from build123d import *

# Parameters (mm, degrees)
F0_W     = 127
F0_H     = 76.2
F1_DEPTH = 25.4
F2_W     = 123.0376
F2_H     = 72.2376
F3_DEPTH = 24.4094
F4_W     = 1.9812
F4_H     = 72.2376
F5_DEPTH = 24.4094
F6_W     = 21.4376
F6_H     = 72.2376
F7_DEPTH = 1.9812


with BuildPart() as f1:
    # F0 (on Front) → F1 (new body)
    with BuildSketch(Plane.XZ):
        Rectangle(F0_W, F0_H)
    extrude(amount=F1_DEPTH)

    # F2 (on Front) → F3 (cut)
    with BuildSketch(Plane.XZ):
        Rectangle(F2_W, F2_H)
    extrude(amount=F3_DEPTH, mode=Mode.SUBTRACT)

    # F4 (on face) → F5 (join)
    with BuildSketch(Plane(origin=(0, -24.4094, 0), x_dir=(-1, 0, 0), z_dir=(0, 1, 0))):
        with Locations((-43.5102, 0)):
            Rectangle(F4_W, F4_H)
    extrude(amount=F5_DEPTH)

    # F6 (on face) → F7 (cut)
    with BuildSketch(Plane(origin=(-63.5, 0, 0), x_dir=(0, -1, 0), z_dir=(-1, 0, 0))):
        with Locations((12.7, 0)):
            Rectangle(F6_W, F6_H)
    extrude(amount=-F7_DEPTH, mode=Mode.SUBTRACT)


solid = f1.part
Could you check a few things on this model? Use its own coordinates, in mm. A direction names the side the tool comes from. Give positions to 0.01 mm unless a question says otherwise; leave off trailing zeros. Order: outer loops, then holes, each group sorted by start corner. A loop starts at its lowest first (then second) coordinate and runs counter-clockwise, first axis right, second up. Notation, with made-up numbers: (79.25, 33) - (103.25, 33) arc R21 cw to (103.25, 60) - close; hole circle Ø1 at (81, 5.25). An arc over 180 degrees is marked (long way). One line per item, written item: value. Start each with the question number.
1. Thinking about a two-plate mould opening in Z: for faces 3 (the face through (-1, -13, -38.1)), 4 (the face through (53, -24.409, 1)), 5 (the face through (0, 0, 37)), 6 (the face through (-1, -13, 38.1)), which applies, +Z half, -Z half, draft (parallel to the pull), parting line (faces both ways), or undercut?
2. If I drill on probe 1 along Z at (x, y) = (-48.5, -19); probe 2 along X at (y, z) = (-11.75, 27); probe 3 along Y at (x, z) = (46.5, -6.5), over which ranges is the centre line in solid material (lowest first)?
3. Imagine slicing it at C-C on x = 36.5. List the corners of the cut face in (y, z) for me, plus the area to 3 significant figures.
4. Imagine slicing it at B-B on y = -20.25. List the corners of the cut face in (x, z) for me, plus the area to 3 significant figures.
5. For P1, Ø3, axis at y = -20.5, z = 15, coming from the -X side; P2, Ø13.5, axis at x = 53, z = -8.5, coming from the +Y side, each with a flat end and sliding along its axis, tell me the tip position at first contact or that it passes through.
6. Imagine slicing it at A-A on z = -27.5. List the corners of the cut face in (x, y) for me.
7. For faces 1 (the face through (-63.5, -24, -3)), 2 (the face through (61.519, -12, -1)), which set-ups out of +Z, -Z, +X, -X, +Y, -Y let a thin tool reach every point of the face, with its end or its side?
Values:
1. face 3: -Z half
1. face 4: undercut
1. face 5: draft
1. face 6: +Z half
2. probe 1: -38.1 to -36.12, 36.12 to 38.1
2. probe 2: 42.52 to 44.5, 61.52 to 63.5
2. probe 3: -25.4 to -24.41
3. outline: (-25.4, -38.1) - (0, -38.1) - (0, -36.12) - (-24.41, -36.12) - (-24.41, 36.12) - (0, 36.12) - (0, 38.1) - (-25.4, 38.1) - close
3. area: 172 mm²
4. outline: (-63.5, -38.1) - (63.5, -38.1) - (63.5, 38.1) - (-63.5, 38.1) - (-63.5, 36.12) - (42.52, 36.12) - (42.52, -36.12) - (-63.5, -36.12) - close; hole (44.5, -36.12) - (61.52, -36.12) - (61.52, 36.12) - (44.5, 36.12) - close
4. area: 789 mm²
5. P1: x = 42.52
5. P2: y = -24.41
6. outline: (-63.5, -25.4) - (63.5, -25.4) - (63.5, 0) - (61.52, 0) - (61.52, -24.41) - (44.5, -24.41) - (44.5, 0) - (42.52, 0) - (42.52, -24.41) - (-61.52, -24.41) - (-61.52, -23.42) - (-63.5, -23.42) - close; (-63.5, -1.98) - (-61.52, -1.98) - (-61.52, 0) - (-63.5, 0) - close
7. face 1: +Z, -Z, -X, +Y, -Y
7. face 2: +Y
